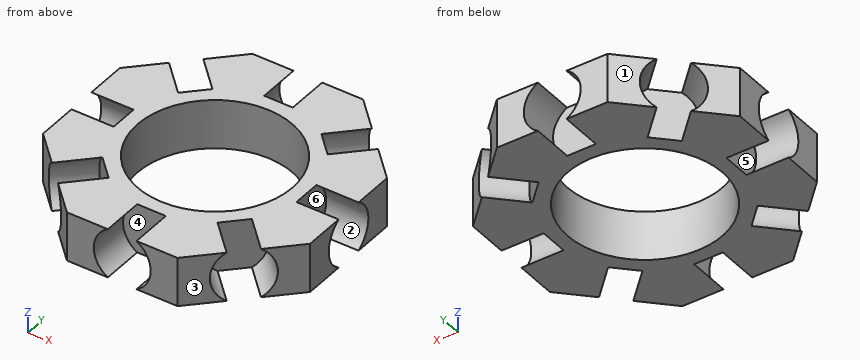
```python
from build123d import *

# Parameters (mm, degrees)
SKETCH1_R           = 11
BOSS_EXTRUDE1_DEPTH = 3.5
SKETCH2_R           = 4.05
CUT_EXTRUDE3_DEPTH  = 6
CIRPATTERN1_COUNT   = 8


with BuildPart() as part:
    # Sketch1 → Boss-Extrude1 (new body, symmetric)
    with BuildSketch(Plane.XY):
        Polygon((7.870057685, 19), (-7.870057685, 19), (-19, 7.870057685), (-19, -7.870057685), (-7.870057685, -19), (7.870057685, -19), (19, -7.870057685), (19, 7.870057685), align=None)
        Circle(SKETCH1_R, mode=Mode.SUBTRACT)
    extrude(amount=BOSS_EXTRUDE1_DEPTH, both=True)

    # Sketch2 → Cut-Extrude3 (cut)
    with BuildSketch(Plane(origin=(0, -19, 0), x_dir=(-1, 0, 0), z_dir=(0, -1, 0))):
        Circle(SKETCH2_R)
    cut_extrude3 = extrude(amount=-CUT_EXTRUDE3_DEPTH, mode=Mode.SUBTRACT)

    # CirPattern1: Cut-Extrude3 ×8 about axis
    cirpattern1_axis = Axis((0, 0, 0), (0, 0, 1))
    for i in range(1, CIRPATTERN1_COUNT):
        add(cut_extrude3.rotate(cirpattern1_axis, i * 360 / CIRPATTERN1_COUNT), mode=Mode.SUBTRACT)


solid = part.part
```
The listing builds one solid part. Answer for the finished solid, in the listing's coordinates (mm). Face numbers are marked on the shaded views. A direction names the side the tool comes from. Coordinates: 2 decimals unless noted, no trailing zeros. Loops run counter-clockwise (first coordinate to the right, second up) from the corner with the lowest first, then second, coordinate; pieces in that order, holes last. Notation, with made-up numbers: (44.5, 31) - (59.5, 31) arc R30 ccw to (59.5, 67) - close; hole circle Ø8 at (11.25, 10.5). An arc over 180 degrees is marked (long way). Write item = value, one per line.
1) Each of these flat-tipped pins is pushed along its axis until it touches: P1, Ø2, axis at y = -9, z = 0, coming from the -X side; P2, Ø4, axis at y = -0.5, z = 2, coming from the -X side; P3, Ø3.5, axis at x = 0, z = 1.5, coming from the -Y side; P4, Ø5, axis at x = -1.5, y = -8, coming from the -Z side. Where does it stop, or does it pass through?
Responses:
P1 = -18.87
P2 = -13
P3 = -13
P4 = through
2) Section B-B (x = 5) is taken. Determine the outline of the cut face in (y, z), plus the area to 3 significant figures.
Responses:
outline = (-19, -3.5) - (-9.8, -3.5) - (-9.8, 3.5) - (-19, 3.5) - close; (9.8, -3.5) - (19, -3.5) - (19, 3.5) - (9.8, 3.5) - close
area = 129 mm^2
3) Which of the six approach directions +Z, -Z, +X, -X, +Y, -Y give full straight-line access (tool end or side, diameter ignored) to the marked faces 4, 5 and 6?
Responses:
face_4 = -Y
face_5 = -X
face_6 = +X
4) Section A-A (y = 0) is taken. Determine the outline of the cut face in (x, z).
Responses:
outline = (-13, -3.5) - (-11, -3.5) - (-11, 3.5) - (-13, 3.5) - close; (11, -3.5) - (13, -3.5) - (13, 3.5) - (11, 3.5) - close
5) Determine the mould class of the marked faces 1, 2 and 3 for opening direction Y: pulls with the +Y half, pulls with the -Y half, needs draft (parallel to the pull), parting line crosses it, or undercut.
Responses:
face_1 = pulls with the +Y half
face_2 = undercut
face_3 = pulls with the -Y half
6) Section C-C (x = -9.5) is taken. Count the separate pieces of the cut face and the enclosed holes in it, plus the area to 3 significant figures.
Responses:
separate_pieces = 4
enclosed_holes = 0
area = 88.3 mm^2
7) Find the intervals of material crossed by line 1 along Y through (x, z) = (0, -0.5); line 2 along Y through (x, z) = (-9, -0.75); line 3 along Y through (x, z) = (7, 2), in increasing order.
Responses:
line_1 = -13 to -11, 11 to 13
line_2 = -17.87 to -14.63, -9.38 to -6.32, 6.32 to 9.38, 14.63 to 17.87
line_3 = -19 to -11.98, -11.38 to -8.49, 8.49 to 11.38, 11.98 to 19
